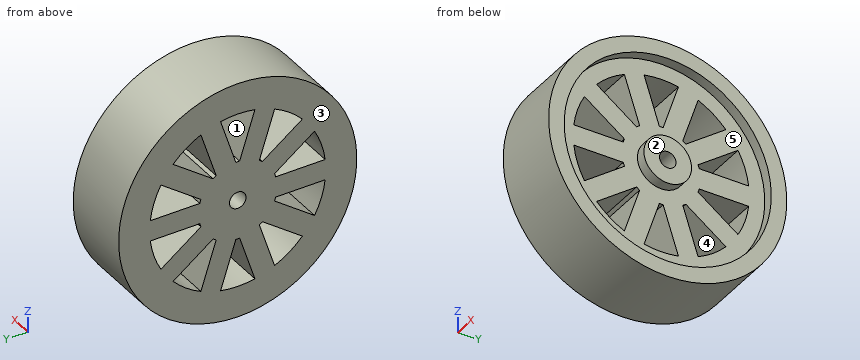
```python
from build123d import *

# Parameters (mm, degrees)
SKETCH1_R               = 29.21
SKETCH1_R_2             = 2.032
BOSS_EXTRUDE1_DEPTH     = 8.89
CUT_EXTRUDE1_DEPTH      = 45.973065272
CUT_EXTRUDE1_DEPTH_BACK = 45.973065272
SKETCH3_R               = 25.4
SKETCH3_R_2             = 5.842
CUT_EXTRUDE2_DEPTH      = 2.54


with BuildPart() as part:
    # Sketch1 → Boss-Extrude1 (new, symmetric)
    with BuildSketch(Plane(origin=(0, 0, 0), x_dir=(0, 0, -1), z_dir=(1, 0, 0))):
        Circle(SKETCH1_R)
        Circle(SKETCH1_R_2, mode=Mode.SUBTRACT)
    extrude(amount=BOSS_EXTRUDE1_DEPTH, both=True)

    # Sketch2 → Cut-Extrude1 (cut, two sides: drawn at the far end of the back side and taken through both)
    with BuildSketch(Plane(origin=(8.89, 0, 0), x_dir=(0, 0, -1), z_dir=(1, 0, 0)).offset(-CUT_EXTRUDE1_DEPTH_BACK)):
        with BuildLine():
            Line((-2.54, 21.44006763), (-2.54, 9.311793812))
            ThreePointArc((-2.54, 9.311793812), (-2.98263203, 9.179597495), (-3.418431909, 9.026373983))
            Line((-3.418431909, 9.026373983), (-10.547252396, 18.838353614))
            ThreePointArc((-10.547252396, 18.838353614), (-6.671676909, 20.533310187), (-2.54, 21.44006763))
        make_face()
        with BuildLine():
            Line((2.54, 21.44006763), (2.54, 9.311793812))
            ThreePointArc((2.54, 9.311793812), (2.98263203, 9.179597495), (3.418431909, 9.026373983))
            Line((3.418431909, 9.026373983), (10.547252396, 18.838353614))
            ThreePointArc((10.547252396, 18.838353614), (6.671676909, 20.533310187), (2.54, 21.44006763))
        make_face()
        with BuildLine():
            Line((14.657058727, 15.852404533), (7.528238241, 6.040424901))
            ThreePointArc((7.528238241, 6.040424901), (7.80863203, 5.673303255), (8.071139018, 5.293186087))
            Line((8.071139018, 5.293186087), (19.605812864, 9.04102881))
            ThreePointArc((19.605812864, 9.04102881), (17.466676909, 12.690283597), (14.657058727, 15.852404533))
        make_face()
        with BuildLine():
            Line((21.175619195, 4.209661707), (9.640945349, 0.461818985))
            ThreePointArc((9.640945349, 0.461818985), (9.652, 0), (9.640945349, -0.461818985))
            Line((9.640945349, -0.461818985), (21.175619195, -4.209661707))
            ThreePointArc((21.175619195, -4.209661707), (21.59, 0), (21.175619195, 4.209661707))
        make_face()
        with BuildLine():
            Line((19.605812864, -9.04102881), (8.071139018, -5.293186087))
            ThreePointArc((8.071139018, -5.293186087), (7.80863203, -5.673303255), (7.528238241, -6.040424901))
            Line((7.528238241, -6.040424901), (14.657058727, -15.852404533))
            ThreePointArc((14.657058727, -15.852404533), (17.466676909, -12.690283597), (19.605812864, -9.04102881))
        make_face()
        with BuildLine():
            Line((10.547252396, -18.838353614), (3.418431909, -9.026373983))
            ThreePointArc((3.418431909, -9.026373983), (2.98263203, -9.179597495), (2.54, -9.311793812))
            Line((2.54, -9.311793812), (2.54, -21.44006763))
            ThreePointArc((2.54, -21.44006763), (6.671676909, -20.533310187), (10.547252396, -18.838353614))
        make_face()
        with BuildLine():
            Line((-2.54, -21.44006763), (-2.54, -9.311793812))
            ThreePointArc((-2.54, -9.311793812), (-2.98263203, -9.179597495), (-3.418431909, -9.026373983))
            Line((-3.418431909, -9.026373983), (-10.547252396, -18.838353614))
            ThreePointArc((-10.547252396, -18.838353614), (-6.671676909, -20.533310187), (-2.54, -21.44006763))
        make_face()
        with BuildLine():
            Line((-14.657058727, -15.852404533), (-7.528238241, -6.040424901))
            ThreePointArc((-7.528238241, -6.040424901), (-7.80863203, -5.673303255), (-8.071139018, -5.293186087))
            Line((-8.071139018, -5.293186087), (-19.605812864, -9.04102881))
            ThreePointArc((-19.605812864, -9.04102881), (-17.466676909, -12.690283597), (-14.657058727, -15.852404533))
        make_face()
        with BuildLine():
            Line((-21.175619195, -4.209661707), (-9.640945349, -0.461818985))
            ThreePointArc((-9.640945349, -0.461818985), (-9.652, 0), (-9.640945349, 0.461818985))
            Line((-9.640945349, 0.461818985), (-21.175619195, 4.209661707))
            ThreePointArc((-21.175619195, 4.209661707), (-21.59, 0), (-21.175619195, -4.209661707))
        make_face()
        with BuildLine():
            Line((-19.605812864, 9.04102881), (-8.071139018, 5.293186087))
            ThreePointArc((-8.071139018, 5.293186087), (-7.80863203, 5.673303255), (-7.528238241, 6.040424901))
            Line((-7.528238241, 6.040424901), (-14.657058727, 15.852404533))
            ThreePointArc((-14.657058727, 15.852404533), (-17.466676909, 12.690283597), (-19.605812864, 9.04102881))
        make_face()
    extrude(amount=CUT_EXTRUDE1_DEPTH + CUT_EXTRUDE1_DEPTH_BACK, mode=Mode.SUBTRACT)

    # Sketch3 → Cut-Extrude2 (cut)
    with BuildSketch(Plane(origin=(8.89, 0, 0), x_dir=(0, 0, -1), z_dir=(1, 0, 0))):
        Circle(SKETCH3_R)
        Circle(SKETCH3_R_2, mode=Mode.SUBTRACT)
    extrude(amount=-CUT_EXTRUDE2_DEPTH, mode=Mode.SUBTRACT)


solid = part.part
```
For this review, take the finished solid that the model builds, in its own axes (mm). Face numbers are marked on the shaded views. A direction names the side the tool comes from. Give positions to 0.01 mm unless a question says otherwise; leave off trailing zeros. Write each loop counter-clockwise with the first axis right and the second up, starting at its lowest first coordinate (ties: lowest second). Pieces come first, ordered by that corner, then holes.
Item 1: Take a section at B-B (z = 11.5). Give the boundary of the cut face in (x, y), and give its area (3 significant figures).
Item 2: Machinability: for the marked faces 3, 4 and 5, which of the approach directions +Z, -Z, +X, -X, +Y, -Y give a long, thin tool a straight path to every point of the face, cutting with its end or side? Answer none if there is none.
Item 3: Wall thickness on probe 1 along Y at (x, z) = (1.75, 0); probe 2 along Z at (x, y) = (6, 16.5); probe 3 along Z at (x, y) = (0, 16): over which ranges is each line inside the solid? List them lowest first.
Item 4: The part is to be moulded in two halves that separate along Y. For the marked faces 1 and 2, say which applies: +Y half, -Y half, draft (parallel to the pull), parting line (faces both ways), or undercut.
Item 5: Take a section at A-A (z = 0). Give the boundary of the cut face in (x, y), and give its area (3 significant figures).
Item 6: Insertion check: P1, Ø1.5, axis at x = -4, z = -6, coming from the -Y side; P2, Ø10, axis at y = -3.5, z = -23.5, coming from the +X side; P3, Ø1, axis at x = -4, z = 11, coming from the +Y side; P4, Ø1.5, axis at x = 1, z = 6, coming from the +Y side. Each pin has a flat end and moves straight along its axis. Give the tip position at first contact, or say it passes through.
Item 7: Take a section at D-D (x = -5.75). Give the number of separate pieces and of enclosed holes in the cut face, and give its area (3 significant figures).
Item 8: Take a section at C-C (y = 13). Give the boundary of the cut face in (x, z).
Established:
1. outline: (-8.89, -26.85) - (8.89, -26.85) - (8.89, -22.65) - (6.35, -22.65) - (6.35, -11.51) - (-8.89, -11.51) - close; (-8.89, -6.41) - (6.35, -6.41) - (6.35, -1.07) - (-8.89, -1.07) - close; (-8.89, 1.07) - (6.35, 1.07) - (6.35, 6.41) - (-8.89, 6.41) - close; (-8.89, 11.51) - (6.35, 11.51) - (6.35, 22.65) - (8.89, 22.65) - (8.89, 26.85) - (-8.89, 26.85) - close
1. area: 652 mm2
2. face 3: +Z, -Z, -X, +Y, -Y
2. face 4: +X, -X
2. face 5: +X
3. probe 1: y = -29.21 to -2.03, 2.03 to 29.21
3. probe 2: z = -24.1 to -8.85, -2.54 to 2.54, 8.85 to 24.1
3. probe 3: z = -24.44 to -8.49, -2.54 to 2.54, 8.49 to 24.44
4. face 1: undercut
4. face 2: draft
5. outline: (-8.89, -29.21) - (8.89, -29.21) - (8.89, -25.4) - (6.35, -25.4) - (6.35, -5.84) - (8.89, -5.84) - (8.89, -2.03) - (-8.89, -2.03) - close; (-8.89, 2.03) - (8.89, 2.03) - (8.89, 5.84) - (6.35, 5.84) - (6.35, 25.4) - (8.89, 25.4) - (8.89, 29.21) - (-8.89, 29.21) - close
5. area: 867 mm2
6. P1: stops at y = -28.73
6. P2: stops at x = 8.89
6. P3: stops at y = 27.26
6. P4: stops at y = 28.73
7. separate pieces: 1
7. enclosed holes: 11
7. area: 2,110 mm2
8. outline: (-8.89, -26.16) - (8.89, -26.16) - (8.89, -21.82) - (6.35, -21.82) - (6.35, -17.24) - (-8.89, -17.24) - close; (-8.89, -12.58) - (6.35, -12.58) - (6.35, -6.31) - (-8.89, -6.31) - close; (-8.89, -2.54) - (6.35, -2.54) - (6.35, 2.54) - (-8.89, 2.54) - close; (-8.89, 6.31) - (6.35, 6.31) - (6.35, 12.58) - (-8.89, 12.58) - close; (-8.89, 17.24) - (6.35, 17.24) - (6.35, 21.82) - (8.89, 21.82) - (8.89, 26.16) - (-8.89, 26.16) - close
